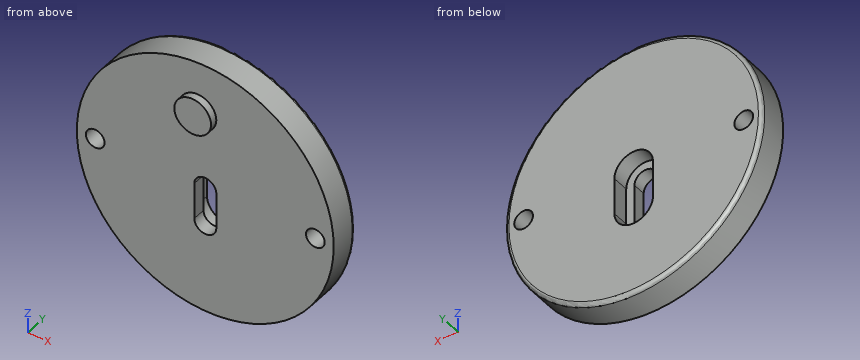
from build123d import *

# Parameters (mm, degrees)
F0_R     = 35
F0_R_2   = 2.55
F0_R_3   = 5
F1_DEPTH = 8
F2_DEPTH = 8
F3_DEPTH = 4.5
F4_R     = 1
F5_DEPTH = 10


with BuildPart() as f1:
    # F0 (on Front) → F1 (new body)
    with BuildSketch(Plane.XZ):
        Circle(F0_R)
        with BuildLine():
            ThreePointArc((-5.25, 0), (0, 5.25), (5.25, 0))
            Line((5.25, 0), (5.25, -10))
            ThreePointArc((5.25, -10), (0, -15.25), (-5.25, -10))
            Line((-5.25, -10), (-5.25, 0))
        make_face(mode=Mode.SUBTRACT)
        with Locations((-30, 0)):
            Circle(F0_R_2, mode=Mode.SUBTRACT)
        with Locations((-2, 20.93092)):
            Circle(F0_R_3, mode=Mode.SUBTRACT)
        with Locations((30, 0)):
            Circle(F0_R_2, mode=Mode.SUBTRACT)
    extrude(amount=F1_DEPTH)

    # F0 (on Front) → F2 (join)
    with BuildSketch(Plane.XZ):
        with BuildLine():
            Line((5.25, -10), (5.25, 0))
            ThreePointArc((5.25, 0), (0, 5.25), (-5.25, 0))
            Line((-5.25, 0), (-5.25, -10))
            ThreePointArc((-5.25, -10), (0, -15.25), (5.25, -10))
        make_face()
        with BuildLine():
            ThreePointArc((-3, 0), (0, 3), (3, 0))
            Line((3, 0), (3, -10))
            ThreePointArc((3, -10), (0, -13), (-3, -10))
            Line((-3, -10), (-3, 0))
        make_face(mode=Mode.SUBTRACT)
    extrude(amount=F2_DEPTH)

    # F0 (on Front) → F3 (cut)
    with BuildSketch(Plane.XZ):
        with BuildLine():
            Line((5.25, -10), (5.25, 0))
            ThreePointArc((5.25, 0), (0, 5.25), (-5.25, 0))
            Line((-5.25, 0), (-5.25, -10))
            ThreePointArc((-5.25, -10), (0, -15.25), (5.25, -10))
        make_face()
        with BuildLine():
            ThreePointArc((-3, 0), (0, 3), (3, 0))
            Line((3, 0), (3, -10))
            ThreePointArc((3, -10), (0, -13), (-3, -10))
            Line((-3, -10), (-3, 0))
        make_face(mode=Mode.SUBTRACT)
    extrude(amount=F3_DEPTH, mode=Mode.SUBTRACT)

    # F4
    f4_edges = [f1.edges().sort_by_distance(p)[0] for p in [
        (-35, 0, 0),
    ]]
    fillet(f4_edges, radius=F4_R)

    # F0 (on Front) → F5 (join)
    with BuildSketch(Plane.XZ):
        with Locations((-2, 20.93092)):
            Circle(F0_R_3)
    extrude(amount=F5_DEPTH)


solid = f1.part
Could you check a few things on this model? Use its own coordinates, in mm. Coordinates: 2 decimals unless noted, no trailing zeros. Order: outer loops, then holes, each group sorted by start corner. A loop starts at its lowest first (then second) coordinate and runs counter-clockwise, first axis right, second up. Notation, with made-up numbers: (36, -33) - (82, -33) arc R19 cw to (82, -20) - close; hole circle Ø9 at (49, 15). An arc over 180 degrees is marked (long way). Answer in a Markdown table with one row per item. Add a question column.
(1) If we section it at A-A, the plane y = -2.25: Please give me the cut outline in (x, z), then the cut area to 3 significant figures.
(2) I need wall thicknesses on L1, parallel to Z at x = 2, y = -5.25; L2, parallel to Z at x = -30.5, y = -7; L3, parallel to Y at x = 28.5, z = 11. Which ranges of each line are inside material? Lowest first, please.
(3) If we section it at C-C, the plane y = -6.25: Please give me the cut outline in (x, z).
(4) If we section it at D-D, the plane z = -1: State how many separate pieces and enclosed holes the cut face has, then the cut area to 3 significant figures.
(5) Will these pins go through, and if not, where does the flat tip stop? pin 1 (1.3 mm diameter, centred on y = -3, z = -6, fed in from -X); pin 2 (1.5 mm diameter, centred on y = -1, z = 12.5, fed in from -X); pin 3 (3 mm diameter, centred on y = -5.5, z = -5, fed in from +X).
(6) If we section it at B-B, the plane x = 0: Please give me the cut outline in (y, z).
Results are:
| question | item | result |
|---|---|---|
| 1 | outline | circle Ø70 at (0, 0); hole circle Ø5.1 at (-30, 0); hole (-5.25, -10) arc R5.25 ccw to (5.25, -10) - (5.25, 0) arc R5.25 ccw to (-5.25, 0) - close; hole circle Ø5.1 at (30, 0) |
| 1 | area | 3,620 mm2 |
| 2 | L1 | z = -34.94 to -12.24, 2.24 to 34.94 |
| 2 | L2 | z = -17.17 to -2.5, 2.5 to 17.17 |
| 2 | L3 | y = -8 to 0 |
| 3 | outline | circle Ø70 at (0, 0); hole circle Ø5.1 at (-30, 0); hole (-3, -10) arc R3 ccw to (3, -10) - (3, 0) arc R3 ccw to (-3, 0) - close; hole circle Ø5.1 at (30, 0) |
| 4 | separate pieces | 4 |
| 4 | enclosed holes | 0 |
| 4 | area | 416 mm2 |
| 5 | pin 1 | stops at x = -34.59 |
| 5 | pin 2 | stops at x = -32.97 |
| 5 | pin 3 | stops at x = 34.82 |
| 6 | outline | (-10, 16.35) - (-8, 16.35) - (-8, 3) - (-4.5, 3) - (-4.5, 5.25) - (0, 5.25) - (0, 34) arc R1 ccw to (-1, 35) - (-8, 35) - (-8, 25.51) - (-10, 25.51) - close; (-8, -35) - (-1, -35) arc R1 ccw to (0, -34) - (0, -15.25) - (-4.5, -15.25) - (-4.5, -13) - (-8, -13) - close |
